from build123d import *

# Parameters (mm, degrees)
F1_DEPTH = 25.4


# Not quite as in the source:
# - a feature names something its author has since deleted; it is built from what else it names


with BuildPart() as f1:
    # F0 (on Front) → F1 (new body)
    with BuildSketch(Plane.XZ):
        Polygon((-41.275, -9.525), (41.275, -9.525), (41.275, 9.525), (22.225, 9.525), (-41.275, 9.525), align=None)
        with BuildLine():
            Line((22.225, 9.525), (41.275, 9.525))
            Line((41.275, 9.525), (41.275, 27.0002))
            ThreePointArc((41.275, 27.0002), (45.9246798487, 38.2255201513), (57.15, 42.8752))
            Line((57.15, 42.8752), (60.325, 42.8752))
            Line((60.325, 42.8752), (60.325, 61.9252))
            Line((60.325, 61.9252), (57.15, 61.9252))
            add(Edge.make_bspline(
                [(57.15, 61.9252), (47.4917497752, 56.7832722029), (37.8334995503, 51.6413444058), (28.1752493255, 46.4994166087)],
                knots=[0, 0, 0, 0, 32.8251575759, 32.8251575759, 32.8251575759, 32.8251575759], degree=3))
            ThreePointArc((28.1752493255, 46.4994166087), (23.7456680032, 37.1936404813), (22.225, 27.0002))
            Line((22.225, 27.0002), (22.225, 9.525))
        make_face()
        with BuildLine():
            add(Edge.make_bspline(
                [(28.1752493255, 46.4994166087), (5.025166217, 34.1746110724), (-18.1249168915, 21.8498055362), (-41.275, 9.525)],
                knots=[32.8251575759, 32.8251575759, 32.8251575759, 32.8251575759, 111.5045361635, 111.5045361635, 111.5045361635, 111.5045361635], degree=3))
            Line((-41.275, 9.525), (22.225, 9.525))
            Line((22.225, 9.525), (22.225, 27.0002))
            ThreePointArc((22.225, 27.0002), (23.7456680032, 37.1936404813), (28.1752493255, 46.4994166087))
        make_face()
        with BuildLine():
            ThreePointArc((57.15, 61.9252), (40.737421212, 57.8284805639), (28.1752493255, 46.4994166087))
            add(Edge.make_bspline(
                [(57.15, 61.9252), (47.4917497752, 56.7832722029), (37.8334995503, 51.6413444058), (28.1752493255, 46.4994166087)],
                knots=[0, 0, 0, 0, 32.8251575759, 32.8251575759, 32.8251575759, 32.8251575759], degree=3))
        make_face()
        Polygon((60.325, 61.9252), (60.325, 42.8752), (60.325, 38.1), (111.125, 38.1), (111.125, 66.675), (60.325, 66.675), align=None)
    extrude(amount=F1_DEPTH)


solid = f1.part
Input: part model. Units: mm. Frame: model coordinates. A direction names the side the tool comes from. Coordinates: 2 decimals unless noted, no trailing zeros. Loops run counter-clockwise (first coordinate to the right, second up) from the corner with the lowest first, then second, coordinate; pieces in that order, holes last. Notation, with made-up numbers: (65.25, 89.25) - (115.25, 89.25) arc R21 ccw to (115.25, 94.25) - close; hole circle Ø11 at (1, -28). An arc over 180 degrees is marked (long way). Answer in a Markdown table with one row per item. Add a question column.
Item 1: Section query B-B on x = 82. Return the cut outline in (y, z) (3 decimals).
Item 2: Line query: line 1 along Z through (x, y) = (84.5, -5.75) (3 decimals); line 2 along X through (y, z) = (-23.5, 40.5) (3 decimals); line 3 along X through (y, z) = (-19.5, -4) (3 decimals). Output: solid intervals per line, ascending. Write a range as [from, to].
Item 3: Access query for faces 1 (the flat face through (41.275, -13, 8)), 2 (the flat face through (60.325, -13, 64)), 3 (the flat face through (60.325, -13, 41)), 4 (the flat face through (111.125, -13, 52)). Directions: +Z, -Z, +X, -X, +Y, -Y. A direction counts if a zero-diameter tool reaches every point of the face in a straight line with its end or side. Return the directions, or none.
Item 4: Mould query, pull axis X, two halves, no side actions, for faces 5 (the flat face through (-41.275, -13, 0)), 6 (the flat face through (85, -13, 38.1)), 7 (the cylindrical face through (45.8, -12.5, 38.1)). Classes: released by +X, released by -X, zero draft, split by the parting line, or undercut.
Item 5: Section query A-A on z = 54. Return the cut outline in (x, y) (3 decimals), then the cut area to 3 significant figures.
Item 6: Contact query for flat-ended pins moving along their axis: P1, Ø3, axis at y = -9.5, z = 17, coming from the +X side (3 decimals); P2, Ø2.5, axis at x = 58, y = -17.5, coming from the +Z side; P3, Ø5, axis at y = -10, z = 41.5, coming from the -X side. Output: stop coordinate, or through.
Recorded:
| question | item | result |
|---|---|---|
| 1 | outline | (-25.4, 38.1) - (0, 38.1) - (0, 66.675) - (-25.4, 66.675) - close |
| 2 | line 1 | [38.1, 66.675] |
| 2 | line 2 | [16.906, 48.797], [60.325, 111.125] |
| 2 | line 3 | [-41.275, 41.275] |
| 3 | face 1 | -Z, +X, +Y, -Y |
| 3 | face 2 | +Z, -X, +Y, -Y |
| 3 | face 3 | -Z, +Y, -Y |
| 3 | face 4 | +Z, -Z, +X, +Y, -Y |
| 4 | face 5 | released by -X |
| 4 | face 6 | zero draft |
| 4 | face 7 | undercut |
| 5 | outline | (34.997, -25.4) - (111.125, -25.4) - (111.125, 0) - (34.997, 0) - close |
| 5 | area | 1,930 mm^2 |
| 6 | P1 | x = 41.275 |
| 6 | P2 | z = 61.93 |
| 6 | P3 | x = 14.09 |
